Geometry check sheet. Reference: the model listing, model coordinates, mm. A direction names the side the tool comes from. Round coordinates to 2 decimals unless told otherwise and drop trailing zeros. Write each loop counter-clockwise with the first axis right and the second up, starting at its lowest first coordinate (ties: lowest second). Pieces come first, ordered by that corner, then holes. Notation, with made-up numbers: (10.5, 85.5) -> (67.5, 85.5) arc R22 ccw to (67.5, 100.5) -> close; hole circle Ø10 at (-15, 8.25). An arc over 180 degrees is marked (long way). One line per question, with ' | ' between items.
```python
from build123d import *

# Parameters (mm, degrees)
SKETCH1_W               = 32
SKETCH1_H               = 30.6
BOSS_EXTRUDE1_DEPTH     = 10
SKETCH3_W               = 32
SKETCH3_H               = 23.6
BOSS_EXTRUDE2_DEPTH     = 10
SKETCH2_W               = 32
SKETCH2_H               = 11.5
BOSS_EXTRUDE3_DEPTH     = 231
SKETCH4_W               = 32
SKETCH4_H               = 13
BOSS_EXTRUDE4_DEPTH     = 10
CUT_EXTRUDE1_DEPTH      = 210.174783375
CUT_EXTRUDE1_DEPTH_BACK = 210.174783375
SKETCH5_R               = 4
SKETCH6_R               = 2
CUT_EXTRUDE2_DEPTH      = 11.5
CUT_EXTRUDE3_DEPTH      = 208


with BuildPart() as part:
    # Sketch1 → Boss-Extrude1 (new body)
    with BuildSketch(Plane(origin=(0, 0, 0), x_dir=(1, 0, 0), z_dir=(0, 1, 0))):
        Rectangle(SKETCH1_W, SKETCH1_H)
    extrude(amount=BOSS_EXTRUDE1_DEPTH)



with BuildPart() as body_2:
    # Sketch3 → Boss-Extrude2 (new body)
    with BuildSketch(Plane(origin=(0, 251, 0), x_dir=(-1, 0, 0), z_dir=(0, -1, 0))):
        with Locations((0, 3.5)):
            Rectangle(SKETCH3_W, SKETCH3_H)
    extrude(amount=BOSS_EXTRUDE2_DEPTH)


with BuildPart() as part_1:
    add(part.part)

    add(body_2.part)  # Boss-Extrude3 merges body 2
    # Sketch2 → Boss-Extrude3 (add)
    with BuildSketch(Plane(origin=(0, 10, 0), x_dir=(1, 0, 0), z_dir=(0, 1, 0))):
        with Locations((0, 9.55)):
            Rectangle(SKETCH2_W, SKETCH2_H)
    extrude(amount=BOSS_EXTRUDE3_DEPTH)

    # Sketch4 → Boss-Extrude4 (add)
    with BuildSketch(Plane(origin=(0, 53, 0), x_dir=(-1, 0, 0), z_dir=(0, -1, 0))):
        with Locations((0, -2.7)):
            Rectangle(SKETCH4_W, SKETCH4_H)
    extrude(amount=BOSS_EXTRUDE4_DEPTH)

    # Sketch5 → Cut-Extrude1 (cut, two sides: drawn at the far end of the back side and taken through both)
    with BuildSketch(Plane.XZ.offset(-43).offset(-CUT_EXTRUDE1_DEPTH_BACK)):
        with Locations(Location((0, 2.7, 0), (0, 0, 270))):
            Circle(SKETCH5_R)
    extrude(amount=CUT_EXTRUDE1_DEPTH + CUT_EXTRUDE1_DEPTH_BACK, mode=Mode.SUBTRACT)

    # Sketch6 → Cut-Extrude2 (cut)
    with BuildSketch(Plane(origin=(0, 0, -15.3), x_dir=(-1, 0, 0), z_dir=(0, 0, -1))):
        with Locations((0, 50.5)):
            Circle(SKETCH6_R)
        with Locations((0, 100.5)):
            Circle(SKETCH6_R)
        with Locations((0, 150.5)):
            Circle(SKETCH6_R)
        with Locations((0, 200.5)):
            Circle(SKETCH6_R)
    extrude(amount=-CUT_EXTRUDE2_DEPTH, mode=Mode.SUBTRACT)

    # Sketch7 → Cut-Extrude3 (cut)
    with BuildSketch(Plane(origin=(0, 251, 0), x_dir=(1, 0, 0), z_dir=(0, 1, 0))):
        with BuildLine():
            Line((-16, 11.85), (-16, 13.45))
            Line((-16, 13.45), (-14.793086969, 13.45))
            ThreePointArc((-14.793086969, 13.45), (-11.7, 12.65), (-14.793086969, 11.85))
            Line((-14.793086969, 11.85), (-16, 11.85))
        make_face()
        with BuildLine():
            Line((14.793086969, 13.45), (16, 13.45))
            Line((16, 13.45), (16, 11.85))
            Line((16, 11.85), (14.793086969, 11.85))
            ThreePointArc((14.793086969, 11.85), (11.7, 12.65), (14.793086969, 13.45))
        make_face()
    extrude(amount=-CUT_EXTRUDE3_DEPTH, mode=Mode.SUBTRACT)


solid = part_1.part
```
(1) Sectioned sample at B-B on y = 107.5. Record the cut outline in (x, z), then the cut area to 3 significant figures.
Resolved:
outline: (-16, -15.3) -> (16, -15.3) -> (16, -13.45) -> (14.79, -13.45) arc R1.65 cw (long way) to (14.79, -11.85) -> (16, -11.85) -> (16, -3.8) -> (-16, -3.8) -> (-16, -11.85) -> (-14.79, -11.85) arc R1.65 cw (long way) to (-14.79, -13.45) -> (-16, -13.45) -> close | area: 347 mm2
(2) Go/stop test with flat-tipped pins: pin 1 (4 mm diameter, centred on x = 3, y = 107.5, fed in from +Z); pin 2 (1 mm diameter, centred on x = -13.5, z = -13.5, fed in from +Y). Record where each tip stops, or that it passes through.
Resolved:
pin 1: stops at z = -3.8 | pin 2: stops at y = 43
(3) Draft check along X on faces 1 (the flat face through (16, 116, -8)), 2 (the flat face through (0, 5, 15.3)), 3 (the cylindrical face through (-2.4, 48.1, 5.9)), 4 (the cylindrical face through (-2.4, 5.1, 5.9)). Enter one of: +X half, -X half, draft (parallel to the pull), parting line (faces both ways), or undercut.
Resolved:
face 1: +X half | face 2: draft | face 3: undercut | face 4: undercut
(4) Sectioned sample at A-A on x = -9.5. Record the cut outline in (y, z), then the cut area to 3 significant figures.
Resolved:
outline: (0, -15.3) -> (251, -15.3) -> (251, 8.3) -> (241, 8.3) -> (241, -3.8) -> (53, -3.8) -> (53, 9.2) -> (43, 9.2) -> (43, -3.8) -> (10, -3.8) -> (10, 15.3) -> (0, 15.3) -> close | area: 3,330 mm2
(5) Access from +Z, -Z, +X, -X, +Y, -Y to the whole of each face (thin tool, end or side, straight path). Record for faces 5 (the cylindrical face through (-2.4, 246.1, 5.9)), 6 (the flat face through (0, 51, -3.8)), 7 (the flat face through (0, 10, 8)), 8 (the flat face through (0, 246, 8.3)).
Resolved:
face 5: +Y, -Y | face 6: -Z | face 7: +Z, +X, -X | face 8: +Z, +X, -X, +Y
(6) Material ranges on line 1 (Y direction, x = 0, z = -9.25); line 2 (Y direction, x = -6.5, z = -3); line 3 (X direction, y = 200.5, z = -12.5), recorded low to high.
Resolved:
line 1: y = 0 to 48.5, 52.5 to 98.5, 102.5 to 148.5, 152.5 to 198.5, 202.5 to 251 | line 2: y = 0 to 10, 43 to 53, 241 to 251 | line 3: x = -11.71 to -2, 2 to 11.71
(7) Sectioned sample at C-C on y = 38.5. Record the cut outline in (x, z), then the cut area to 3 significant figures.
Resolved:
outline: (-16, -15.3) -> (16, -15.3) -> (16, -3.8) -> (-16, -3.8) -> close | area: 368 mm2
